Input: part model. Units: mm. Frame: model coordinates. Face numbers are marked on the shaded views. Round coordinates to 2 decimals unless told otherwise and drop trailing zeros. Loops run counter-clockwise (first coordinate to the right, second up) from the corner with the lowest first, then second, coordinate; pieces in that order, holes last. Notation, with made-up numbers: (-17.75, 14) - (18.25, 14) arc R21 ccw to (18.25, 18) - close; hole circle Ø11 at (22, -33.5). An arc over 180 degrees is marked (long way). Use CSV: the item, a comma, the result in double quotes. Start each with the question number.
1. Pin query (flat end, axial travel): P1, Ø12, axis at x = 93, z = -79.5, coming from the +Y side; P2, Ø2, axis at x = -16, y = 4, coming from the -Z side. Return the tip coordinate at first contact, or that it passes through.
2. Material intervals for probe 1 along X at (y, z) = (11.75, -184.5); probe 2 along Y at (x, z) = (-71.5, -100); probe 3 along X at (y, z) = (1, -70), sorted ascending. Write a range as from..to.
3. Cut plane B-B (z = -105). Return loops of the section in (x, y).
4. Cut plane C-C (x = -70). Return loops of the section in (y, z), and give its area (3 significant figures).
5. Pull-direction query (X, two-part tool) for the marked faces 1 and 2; classes: +X half, -X half, draft (parallel to the pull), parting line (faces both ways), or undercut.
6. Cut plane A-A (y = 6.25). Return loops of the section in (x, z).
Autodesk Inventor part; units mm, degrees
ref_plane "YZ Plane" through (0, 0, 0) normal (1, 0, 0) x (0, 1, 0)
ref_plane "XZ Plane" through (0, 0, 0) normal (0, 1, 0) x (-1, 0, 0)
ref_plane "XY Plane" through (0, 0, 0) normal (0, 0, 1) x (1, 0, 0)
sketch "Sketch1" plane through (0, 0, 0) normal (0, 1, 0) x (-1, 0, 0)
  line L0 (0, 0) -> (150, 0)
  line L1 (150, 0) -> (150, -200)
  line L2 (150, -200) -> (0, -200)
  line L3 (0, -200) -> (0, 0)
  dimension "d0" = 150
  dimension "d1" = 200
extrude "Plate1" add sketch "Sketch1" along normal blind 1.5
sketch "Sketch2" plane through (-150, 1.5, 0) normal (-1, 0, 0) x (0, -1, 0)
  line L0 (0, -200) -> (0, 0)
  line L1 (0, 0) -> (-18.5, 0)
  line L2 (-18.5, 0) -> (-18.5, -200)
  line L3 (-18.5, -200) -> (0, -200)
edge flange "Flange1" height 20 angle 90 thickness 1.5 bend radius 1.5 thickness toward (-1, 0, 0) relief tear relief width 1.5 relief depth 0.75 edges at (-150, 1.5, -100) wall of the first edge with corners at (-150, 1.5, -200) (-150, 1.5, 0) (-150, 20, 0) (-150, 20, -200)
bend "Bend1"
corner "Corner1"
mirror "Mirror1" about plane through (0, 0, -200) normal (1, 0, 0)
equation "\"d2\" = Thickness"
equation "\"d3\" = BendReliefWidth"
equation "\"d4\" = BendReliefDepth"
equation "\"d5\" = MinimumRemnant"
equation "\"d6\" = TransitionRadius"
equation "\"d9\" = BendRadius"
equation "\"d10\" = CornerReliefSize"
equation "\"d11\" = GapSize"
equation "\"d12\" = JacobiRadiusSize"
equation "\"BendRadius\" = Thickness"
equation "\"BendReliefWidth\" = Thickness"
equation "\"BendReliefDepth\" = 0.5 * Thickness"
equation "\"CornerReliefSize\" = 4 * Thickness"
equation "\"MinimumRemnant\" = 2 * Thickness"
equation "\"TransitionRadius\" = BendRadius"
equation "\"JacobiRadiusSize\" = BendRadius"
equation "\"GapSize\" = Thickness"
properties part number "Magazine bottom"
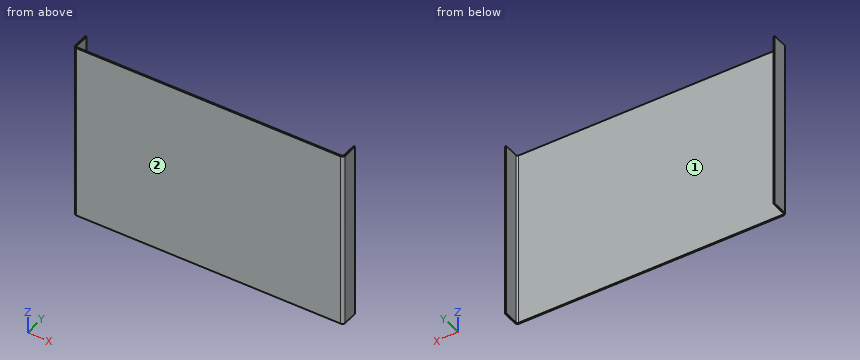
Established:
1,P1,"stops at y = 1.5"
1,P2,"passes through"
2,probe 1,"x = -151.5..-150, 150..151.5"
2,probe 2,"y = 0..1.5"
2,probe 3,"x = -150.74..150.74"
3,outline,"(-151.5, 3) arc R3 ccw to (-148.5, 0) - (148.5, 0) arc R3 ccw to (151.5, 3) - (151.5, 20) - (150, 20) - (150, 3) arc R1.5 cw to (148.5, 1.5) - (-148.5, 1.5) arc R1.5 cw to (-150, 3) - (-150, 20) - (-151.5, 20) - close"
4,outline,"(0, -200) - (1.5, -200) - (1.5, 0) - (0, 0) - close"
4,area,"300 mm2"
5,face 1,"undercut"
5,face 2,"draft"
6,outline,"(-151.5, -200) - (-150, -200) - (-150, 0) - (-151.5, 0) - close; (150, -200) - (151.5, -200) - (151.5, 0) - (150, 0) - close"
